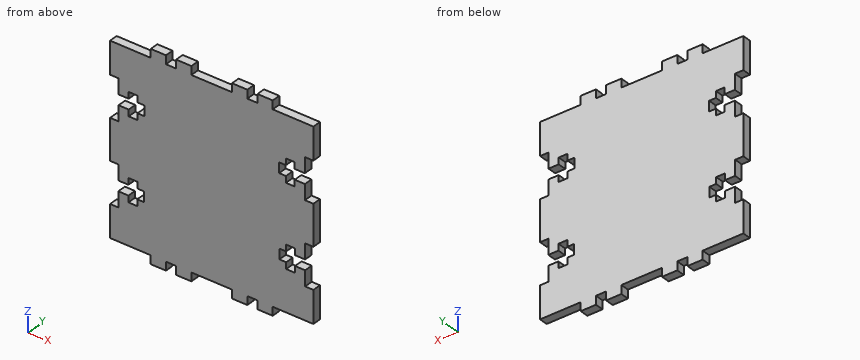
```python
from build123d import *

# Parameters (mm, degrees)
BOSS_EXTRUDE1_DEPTH = 3.175


with BuildPart() as part:
    # Sketch1 → Boss-Extrude1 (new body)
    with BuildSketch(Plane(origin=(0, 0, 0), x_dir=(1, 0, 0), z_dir=(0, 1, 0))):
        Polygon((-27.813, -13.335), (-25.273, -13.335), (-25.273, -17.145), (-27.813, -17.145), (-27.813, -19.558), (-31.115, -19.558), (-31.115, -17.145), (-34.925, -17.145), (-34.925, -22.86), (-38.1, -22.86), (-38.1, -34.925), (-34.925, -34.925), (-22.86, -34.925), (-22.86, -38.1), (-17.145, -38.1), (-17.145, -34.925), (-13.335, -34.925), (-13.335, -38.1), (-7.62, -38.1), (-7.62, -34.925), (7.62, -34.925), (7.62, -38.1), (13.335, -38.1), (13.335, -34.925), (17.145, -34.925), (17.145, -38.1), (22.86, -38.1), (22.86, -34.925), (34.925, -34.925), (38.1, -34.925), (38.1, -22.86), (34.925, -22.86), (34.925, -17.145), (31.115, -17.145), (31.115, -19.558), (27.813, -19.558), (27.813, -17.145), (25.273, -17.145), (25.273, -13.335), (27.813, -13.335), (27.813, -10.922), (31.115, -10.922), (31.115, -13.335), (34.925, -13.335), (34.925, -7.62), (38.1, -7.62), (38.1, 7.62), (35.021495431, 7.62), (35.021495431, 13.335), (31.211495431, 13.335), (31.211495431, 10.922), (27.909495431, 10.922), (27.909495431, 13.335), (25.369495431, 13.335), (25.369495431, 17.145), (27.909495431, 17.145), (27.909495431, 19.558), (31.211495431, 19.558), (31.211495431, 17.145), (35.021495431, 17.145), (35.021495431, 22.86), (38.1, 22.86), (38.1, 34.925), (34.925, 34.925), (22.86, 34.925), (22.86, 38.1), (17.145, 38.1), (17.145, 34.925), (13.335, 34.925), (13.335, 38.1), (7.62, 38.1), (7.62, 34.925), (-7.62, 34.925), (-7.62, 38.1), (-13.335, 38.1), (-13.335, 34.925), (-17.145, 34.925), (-17.145, 38.1), (-22.86, 38.1), (-22.86, 34.925), (-34.925, 34.925), (-38.1, 34.925), (-38.1, 22.86), (-35.021495431, 22.86), (-35.021495431, 17.145), (-31.211495431, 17.145), (-31.211495431, 19.558), (-27.909495431, 19.558), (-27.909495431, 17.145), (-25.369495431, 17.145), (-25.369495431, 13.335), (-27.909495431, 13.335), (-27.909495431, 10.922), (-31.211495431, 10.922), (-31.211495431, 13.335), (-35.021495431, 13.335), (-35.021495431, 7.62), (-38.1, 7.62), (-38.1, -7.62), (-34.925, -7.62), (-34.925, -13.335), (-31.115, -13.335), (-31.115, -10.922), (-27.813, -10.922), align=None)
    extrude(amount=BOSS_EXTRUDE1_DEPTH)


solid = part.part
```
Work out the finished part from the listing and answer in its coordinate system (mm). Round coordinates to 2 decimals unless told otherwise and drop trailing zeros. Loops run counter-clockwise (first coordinate to the right, second up) from the corner with the lowest first, then second, coordinate; pieces in that order, holes last. Notation, with made-up numbers: (57, 84.5) -> (97, 84.5) arc R27 ccw to (97, 107.5) -> close; hole circle Ø4 at (79, 47.5). An arc over 180 degrees is marked (long way). Write each question's results on one line, items separated by ' | '. Start each with the question number.
1. Section C-C (x = 0.5) is taken. Determine the outline of the cut face in (y, z) (3 decimals).
2. Section A-A (x = 29) is taken. Determine the outline of the cut face in (y, z) (3 decimals), plus the area to 3 significant figures.
3. Given pin 1 Ø1.6 at (x, y) = (33.5, 2) entering from -Z (3 decimals); pin 2 Ø5 at (x, z) = (22, 20.5) entering from -Y; pin 3 Ø0.7 at (y, z) = (2, -19) entering from +X; pin 4 Ø1.2 at (y, z) = (2.5, 12) entering from +X (3 decimals), each flat-ended and moving along its own axis, determine where each tip first touches the part or whether it passes through.
4. Find the intervals of material crossed by probe 1 along X at (y, z) = (2.3, 13) (3 decimals); probe 2 along Z at (x, y) = (26, 0.8) (3 decimals); probe 3 along X at (y, z) = (2.45, 35) (3 decimals), in increasing order. Write a range as from..to.
5. Section B-B (z = -9) is taken. Determine the outline of the cut face in (x, y) (1 decimal), plus the area to 3 significant figures.
Evaluation:
1) outline: (0, -34.925) -> (3.175, -34.925) -> (3.175, 34.925) -> (0, 34.925) -> close
2) outline: (0, -34.925) -> (3.175, -34.925) -> (3.175, -19.558) -> (0, -19.558) -> close; (0, -10.922) -> (3.175, -10.922) -> (3.175, 10.922) -> (0, 10.922) -> close; (0, 19.558) -> (3.175, 19.558) -> (3.175, 34.925) -> (0, 34.925) -> close | area: 167 mm2
3) pin 1: stops at z = -34.925 | pin 2: stops at y = 0 | pin 3: stops at x = 35.02 | pin 4: stops at x = 34.925
4) probe 1: x = -34.925..-31.115, -27.813..27.813, 31.115..34.925 | probe 2: z = -34.925..-17.145, -13.335..13.335, 17.145..34.925 | probe 3: x = -22.86..-17.145, -13.335..-7.62, 7.62..13.335, 17.145..22.86
5) outline: (-35, 0) -> (35, 0) -> (35, 3.2) -> (-35, 3.2) -> close | area: 222 mm2
